The listing builds one solid part. Answer for the finished solid, in the listing's coordinates (mm). Give positions to 0.01 mm unless a question says otherwise; leave off trailing zeros. Write each loop counter-clockwise with the first axis right and the second up, starting at its lowest first coordinate (ties: lowest second). Pieces come first, ordered by that corner, then holes. Notation, with made-up numbers: M 52.5,38.25 L 102.5,38.25 A19 ccw 102.5,48.25 Z; hole C 13.5,79.5 d1. An arc over 180 degrees is marked long. Return JSON: item names as keys, results as strings.
from build123d import *

# Parameters (mm, degrees)
BOSS_EXTRUDE1_DEPTH = 10
SKETCH2_R           = 12.7
CUT_EXTRUDE1_DEPTH  = 10
FILLET1_R           = 40


with BuildPart() as part:
    # Sketch1 → Boss-Extrude1 (new body)
    with BuildSketch(Plane(origin=(0, 0, 0), x_dir=(1, 0, 0), z_dir=(0, 1, 0))):
        Polygon((-63.639610307, 148.492424049), (148.492424049, -63.639610307), (63.639610307, -148.492424049), (-148.492424049, 63.639610307), align=None)
    extrude(amount=BOSS_EXTRUDE1_DEPTH)

    # Sketch2 → Cut-Extrude1 (cut)
    with BuildSketch(Plane(origin=(0, 10, 0), x_dir=(1, 0, 0), z_dir=(0, 1, 0))):
        with Locations(Location((-84.852813742, 84.852813742, 0), (0, 0, 270))):
            Circle(SKETCH2_R)
        with Locations(Location((84.852813742, -84.852813742, 0), (0, 0, 270))):
            Circle(SKETCH2_R)
    extrude(amount=-CUT_EXTRUDE1_DEPTH, mode=Mode.SUBTRACT)

    # Fillet1
    fillet1_edges = [part.edges().sort_by_distance(p)[0] for p in [
        (148.492424049, 5, 63.639610307),
        (63.639610307, 5, 148.492424049),
        (-148.492424049, 5, -63.639610307),
        (-63.639610307, 5, -148.492424049),
    ]]
    fillet(fillet1_edges, radius=FILLET1_R)


solid = part.part
Item 1: A cutting plane is placed at A-A, the plane y = 8. Write down the section's boundary in (x, z), plus the area to 3 significant figures.
Geometry results:
{"outline": "M -120.21,-91.92 L -91.92,-120.21 A40 ccw -35.36,-120.21 L 120.21,35.36 A40 ccw 120.21,91.92 L 91.92,120.21 A40 ccw 35.36,120.21 L -120.21,-35.36 A40 ccw Z; hole C -84.85,-84.85 d25.4; hole C 84.85,84.85 d25.4", "area": "33,600 mm2"}
Item 2: Find the intervals of material crossed by line 1 (X direction, y = 1, z = 92); line 2 (X direction, y = 7.25, z = 89.5); line 3 (Z direction, x = 83.5, y = 6.25), in increasing order.
Geometry results:
{"line 1": "x = 7.15 to 74.35, 95.35 to 120.13", "line 2": "x = 4.65 to 73.03, 96.67 to 122.44", "line 3": "z = -1.35 to 72.23, 97.48 to 126.65"}
Item 3: Given pin 1 Ø6 at (y, z) = (4, 99) entering from +X; pin 2 Ø23 at (x, z) = (84.85, 84.85) entering from +Y; pin 3 Ø1 at (y, z) = (7, -86) entering from -X; pin 4 Ø5 at (y, z) = (3.5, 100.5) entering from +X, each flat-ended and moving along its own axis, determine where each tip first touches the part or whether it passes through.
Geometry results:
{"pin 1": "stops at x = 116.13", "pin 2": "passes through", "pin 3": "stops at x = -125.42", "pin 4": "stops at x = 114.13"}
Item 4: A cutting plane is placed at C-C, the plane z = 8.5. Write down the section's boundary in (x, y).
Geometry results:
{"outline": "M -76.35,0 L 93.35,0 L 93.35,10 L -76.35,10 Z"}
Item 5: A cutting plane is placed at B-B, the plane x = 11.5. Write down the section's boundary in (y, z).
Geometry results:
{"outline": "M 0,-73.35 L 10,-73.35 L 10,96.35 L 0,96.35 Z"}
Item 6: Determine the mould class of faces 1 (the cylindrical face through (64.08, 5.07, 131.92)), 2 (the flat face through (2, 10, -2)), 3 (the cylindrical face through (-72.26, 5.07, -86.51)) for opening direction X: +X half, -X half, draft (parallel to the pull), parting line (faces both ways), or undercut.
Geometry results:
{"face 1": "parting line", "face 2": "draft", "face 3": "undercut"}
